from build123d import *

# Parameters (mm, degrees)
SKETCH1_W           = 10
SKETCH1_H           = 10
BOSS_EXTRUDE1_DEPTH = 10
SKETCH3_R           = 1
CUT_EXTRUDE1_DEPTH  = 1
SKETCH4_W           = 1
SKETCH4_H           = 2
CUT_EXTRUDE2_DEPTH  = 0.5
SKETCH5_R           = 0.75
CUT_EXTRUDE3_DEPTH  = 0.5


with BuildPart() as part:
    # Sketch1 → Boss-Extrude1 (new body)
    with BuildSketch(Plane.XY):
        with Locations((5, 5)):
            Rectangle(SKETCH1_W, SKETCH1_H)
    extrude(amount=-BOSS_EXTRUDE1_DEPTH)

    # Sketch3 → Cut-Extrude1 (cut)
    with BuildSketch(Plane(origin=(0, 0, -3), x_dir=(-1, 0, 0), z_dir=(0, 0, -1))):
        with Locations((-8.022028726, 7.600171924)):
            Circle(SKETCH3_R)
    extrude(amount=-CUT_EXTRUDE1_DEPTH, mode=Mode.SUBTRACT)

    # Sketch4 → Cut-Extrude2 (cut)
    with BuildSketch(Plane.XY):
        with Locations((2.017763854, 2.01343797)):
            Rectangle(SKETCH4_W, SKETCH4_H)
    extrude(amount=-CUT_EXTRUDE2_DEPTH, mode=Mode.SUBTRACT)

    # Sketch5 → Cut-Extrude3 (cut)
    with BuildSketch(Plane.XY):
        with Locations((7.070933391, 8.551267259)):
            Circle(SKETCH5_R)
    extrude(amount=-CUT_EXTRUDE3_DEPTH, mode=Mode.SUBTRACT)


solid = part.part
For this review, take the finished solid that the model builds, in its own axes (mm). A direction names the side the tool comes from. Round coordinates to 2 decimals unless told otherwise and drop trailing zeros. Loops run counter-clockwise (first coordinate to the right, second up) from the corner with the lowest first, then second, coordinate; pieces in that order, holes last. Notation, with made-up numbers: (34.5, 69.5) - (61.5, 69.5) arc R12 cw to (61.5, 88.5) - close; hole circle Ø3 at (5, -7). An arc over 180 degrees is marked (long way). Put each result on its own line as item: value. Start each with the question number.
1. Mouldability with a two-part tool opening along Z and no side actions: class faces 1 (the flat face through (8, 8, -2)), 2 (the flat face through (5, 10, -5)), 3 (the flat face through (5, 5, -10)) as +Z half, -Z half, draft (parallel to the pull), parting line (faces both ways), or undercut.
2. Consider section A-A on y = 8. State the section outline as (x, z) points, plus the area to 3 significant figures.
3. Insertion check: P1, Ø6, axis at x = 6.5, z = -4.5, coming from the -Y side; P2, Ø0.8, axis at x = 7, y = 8.5, coming from the +Z side. Each pin has a flat end and moves straight along its axis. Give the tip position at first contact, or say it passes through.
4. For faces 4 (the flat face through (8, 8, -3)), 5 (the flat face through (2, 2, -0.5)), 6 (the flat face through (5, 0, -5)), list the 3-axis set-ups (+Z, -Z, +X, -X, +Y, -Y) from which the entire face can be reached by the end or side of a thin tool; tool diameter is ignored.
5. For probe 1 along Z at (x, y) = (2, 1.75); probe 2 along Y at (x, z) = (7.75, -2.5); probe 3 along Y at (x, z) = (7.75, -0.25), list the stretches that pass through material, from the lowest coordinate up. Write a range as [from, to].
6. Consider section C-C on z = -2.25. State the section outline as (x, y) points, plus the area to 3 significant figures.
7. Consider section B-B on x = 7.25. State the section outline as (y, z) points.
Result sheet:
1. face 1: undercut
1. face 2: draft
1. face 3: -Z half
2. outline: (0, -10) - (10, -10) - (10, 0) - (7.58, 0) - (7.58, -0.5) - (6.56, -0.5) - (6.56, 0) - (0, 0) - close; hole (7.11, -3) - (8.94, -3) - (8.94, -2) - (7.11, -2) - close
2. area: 97.7 mm^2
3. P1: y = 0
3. P2: z = -0.5
4. face 4: none
4. face 5: +Z
4. face 6: +Z, -Z, +X, -X, -Y
5. probe 1: [-10, -0.5]
5. probe 2: [0, 6.64], [8.56, 10]
5. probe 3: [0, 8.23], [8.87, 10]
6. outline: (0, 0) - (10, 0) - (10, 10) - (0, 10) - close; hole circle Ø2 at (8.02, 7.6)
6. area: 96.9 mm^2
7. outline: (0, -10) - (10, -10) - (10, 0) - (9.28, 0) - (9.28, -0.5) - (7.82, -0.5) - (7.82, 0) - (0, 0) - close; hole (6.96, -3) - (8.24, -3) - (8.24, -2) - (6.96, -2) - close
